from build123d import *

# Parameters (mm, degrees)
SKETCH1_W                                           = 260
SKETCH1_H                                           = 190
BOSS_EXTRUDE1_DEPTH                                 = 40
SKETCH2_R                                           = 22
CUT_EXTRUDE1_DEPTH                                  = 166.90660023
M24X2_0_TAPPED_HOLE1_D                              = 22
SKETCH7_W                                           = 70.1
SKETCH7_H                                           = 55.1
CUT_EXTRUDE2_DEPTH                                  = 20
SKETCH8_R                                           = 5
CUT_EXTRUDE3_DEPTH                                  = 20
CBORE_FOR_M8_HEX_SOCKET_HEAD_CAP_SCREW1_D           = 8.4
CBORE_FOR_M8_HEX_SOCKET_HEAD_CAP_SCREW1_CBORE_D     = 15
CBORE_FOR_M8_HEX_SOCKET_HEAD_CAP_SCREW1_CBORE_DEPTH = 8.6
F_8_0MM_DOWEL_HOLE1_D                               = 8


with BuildPart() as part:
    # Sketch1 → Boss-Extrude1 (new body)
    with BuildSketch(Plane(origin=(0, 0, 0), x_dir=(1, 0, 0), z_dir=(0, 1, 0))):
        Rectangle(SKETCH1_W, SKETCH1_H)
    extrude(amount=-BOSS_EXTRUDE1_DEPTH)

    # Sketch2 → Cut-Extrude1 (cut, through all)
    with BuildSketch(Plane(origin=(0, 0, 0), x_dir=(1, 0, 0), z_dir=(0, 1, 0))):
        with Locations(Location((-90, 55, 0), (0, 0, 270))):
            Circle(SKETCH2_R)
        with Locations(Location((90, 55, 0), (0, 0, 270))):
            Circle(SKETCH2_R)
    extrude(amount=-CUT_EXTRUDE1_DEPTH, mode=Mode.SUBTRACT)

    # M24x2.0 Tapped Hole1 (through all)
    with Locations(Plane(origin=(0, 0, 0), x_dir=(1, 0, 0), z_dir=(0, 1, 0))):
        with Locations((0, -32.5)):
            Hole(M24X2_0_TAPPED_HOLE1_D / 2)

    # Sketch7 → Cut-Extrude2 (cut)
    with BuildSketch(Plane(origin=(0, -40, 0), x_dir=(1, 0, 0), z_dir=(0, 1, 0))):
        with Locations((0, -32.5)):
            Rectangle(SKETCH7_W, SKETCH7_H)
    extrude(amount=CUT_EXTRUDE2_DEPTH, mode=Mode.SUBTRACT)

    # Sketch8 → Cut-Extrude3 (cut)
    with BuildSketch(Plane.XZ.offset(40)):
        with Locations((-35.05, 60.05)):
            Circle(SKETCH8_R)
        with Locations((35.05, 60.05)):
            Circle(SKETCH8_R)
        with Locations((-35.05, 4.95)):
            Circle(SKETCH8_R)
        with Locations((35.05, 4.95)):
            Circle(SKETCH8_R)
    extrude(amount=-CUT_EXTRUDE3_DEPTH, mode=Mode.SUBTRACT)

    # CBORE for M8 Hex Socket Head Cap Screw1 (through all)
    with Locations(Plane(origin=(0, 0, 0), x_dir=(1, 0, 0), z_dir=(0, 1, 0))):
        with Locations((-75, -71), (-75, 6), (75, 6), (75, -71)):
            CounterBoreHole(CBORE_FOR_M8_HEX_SOCKET_HEAD_CAP_SCREW1_D / 2, CBORE_FOR_M8_HEX_SOCKET_HEAD_CAP_SCREW1_CBORE_D / 2, CBORE_FOR_M8_HEX_SOCKET_HEAD_CAP_SCREW1_CBORE_DEPTH)

    # Ø8.0mm Dowel Hole1 (through all)
    with Locations(Plane(origin=(0, 0, 0), x_dir=(1, 0, 0), z_dir=(0, 1, 0))):
        with Locations((-75, -32.5), (75, -32.5)):
            Hole(F_8_0MM_DOWEL_HOLE1_D / 2)


solid = part.part
Verification items for the finished model (mm, model axes). A direction names the side the tool comes from. Round coordinates to 2 decimals unless told otherwise and drop trailing zeros. Loops run counter-clockwise (first coordinate to the right, second up) from the corner with the lowest first, then second, coordinate; pieces in that order, holes last. Notation, with made-up numbers: (14.25, -35.75) - (43.25, -35.75) arc R11 cw to (43.25, -26.75) - close; hole circle Ø4 at (-25.75, 80.5). An arc over 180 degrees is marked (long way). Use a Markdown table: item, result. Add a question column.
1. Gauge pin test, flat ends, axial feed: pin 1 (9.5 mm diameter, centred on x = 75, z = 71, fed in from +Y); pin 2 (9 mm diameter, centred on x = 35.05, z = 4.95, fed in from -Y). Record the tip position at first contact, or that the pin passes through.
2. Access from +Z, -Z, +X, -X, +Y, -Y to the whole of each face (thin tool, end or side, straight path). Record for faces 4 (the face through (-2, -20, 95)), 5 (the face through (-71.8, -8.6, 74.2)), 6 (the face through (0, -30, 4.95)).
3. Section check D-D, the plane x = 27. Record the boundary of the cut face in (y, z).
4. Release check for a two-part mould opening along Z. For faces 1 (the face through (-82.493, -4.24, 70.67)), 2 (the face through (-2, -20, -95)), 3 (the face through (130, -20, 1)) record: released by +Z, released by -Z, zero draft, split by the parting line, or undercut.
5. Thickness scan on probe 1 along X at (y, z) = (-7, -56); probe 2 along X at (y, z) = (-29, 71); probe 3 along Z at (x, y) = (75, -19). Record the ranges inside material, lowest first. Write a range as [from, to].
6. Section check A-A, the plane z = -6. Record the boundary of the cut face in (x, y), plus the area to 3 significant figures.
7. Section check C-C, the plane z = -55. Record the boundary of the cut face in (x, y), plus the area to 3 significant figures.
8. Section check B-B, the plane x = 90. Record the boundary of the cut face in (y, z).
Checks:
| question | item | result |
|---|---|---|
| 1 | pin 1 | stops at y = -8.6 |
| 1 | pin 2 | stops at y = -20 |
| 2 | face 4 | +Z, +X, -X, +Y, -Y |
| 2 | face 5 | +Y |
| 2 | face 6 | -Y |
| 3 | outline | (-40, -95) - (0, -95) - (0, 95) - (-40, 95) - (-40, 60.05) - (-20, 60.05) - (-20, 4.95) - (-40, 4.95) - close |
| 4 | face 1 | undercut |
| 4 | face 2 | released by -Z |
| 4 | face 3 | zero draft |
| 5 | probe 1 | x = [-130, -111.98], [-68.02, 68.02], [111.98, 130] |
| 5 | probe 2 | x = [-130, -79.2], [-70.8, 70.8], [79.2, 130] |
| 5 | probe 3 | z = [-95, -71.09], [-38.91, -10.2], [-1.8, 28.5], [36.5, 66.8], [75.2, 95] |
| 6 | outline | (-130, -40) - (-79.2, -40) - (-79.2, -8.6) - (-82.5, -8.6) - (-82.5, 0) - (-130, 0) - close; (-70.8, -40) - (70.8, -40) - (70.8, -8.6) - (67.5, -8.6) - (67.5, 0) - (-67.5, 0) - (-67.5, -8.6) - (-70.8, -8.6) - close; (79.2, -40) - (130, -40) - (130, 0) - (82.5, 0) - (82.5, -8.6) - (79.2, -8.6) - close |
| 6 | area | 9,610 mm^2 |
| 7 | outline | (-130, -40) - (-112, -40) - (-112, 0) - (-130, 0) - close; (-68, -40) - (68, -40) - (68, 0) - (-68, 0) - close; (112, -40) - (130, -40) - (130, 0) - (112, 0) - close |
| 7 | area | 6,880 mm^2 |
| 8 | outline | (-40, -95) - (0, -95) - (0, -77) - (-40, -77) - close; (-40, -33) - (0, -33) - (0, 95) - (-40, 95) - close |
